Work out the finished part from the listing and answer in its coordinate system (mm). A direction names the side the tool comes from. Give positions to 0.01 mm unless a question says otherwise; leave off trailing zeros. Write each loop counter-clockwise with the first axis right and the second up, starting at its lowest first coordinate (ties: lowest second). Pieces come first, ordered by that corner, then holes.
1) A tool of negligible diameter and unlimited length cuts with its end or side. For faces 4 (the face through (9.1, 3.4, -3.3)), 5 (the face through (-0.1, 8.3, 6.2)), from which of +Z, -Z, +X, -X, +Y, -Y can it reach the whole face along a straight path? Write none if from no direction.
2) Find section D-D (x = 6.5). Determine the outline of the cut face in (y, z), plus the area to 3 significant figures.
3) Find section B-B (z = 0). Determine the outline of the cut face in (x, y) (3 decimals), plus the area to 3 significant figures.
4) Straight lines are drawn through the part: probe 1 along Z at (x, y) = (0, 6.5) (3 decimals); probe 2 along Y at (x, z) = (12.75, -2.25); probe 3 along X at (y, z) = (4, -0.75). For each, find the intervals that lie inside material, in ascending order.
5) Find section A-A (x = 0). Determine the outline of the cut face in (y, z) (3 decimals).
6) Determine the mould class of faces 1 (the face through (3, 0, 6)), 2 (the face through (-6, 4, 0)), 3 (the face through (-7.559, 5.816, 5.796)) for opening direction Z: pulls with the +Z half, pulls with the -Z half, needs draft (parallel to the pull), parting line crosses it, or undercut.
7) Given pin 1 Ø4 at (y, z) = (3, 5) entering from +X; pin 2 Ø5 at (x, z) = (1, -0.5) entering from +Y; pin 3 Ø3 at (x, z) = (-3, 11) entering from -Y; pin 4 Ø4 at (y, z) = (3.5, -6.5) entering from -X, each flat-ended and moving along its own axis, determine where each tip first touches the part or whether it passes through.
8) Find section C-C (y = 1.25). Determine the outline of the cut face in (x, z).
```python
from build123d import *

# Parameters (mm, degrees)
SKETCH1_R           = 13.9
BOSS_EXTRUDE1_DEPTH = 3.4
SKETCH2_R           = 9.525
BOSS_EXTRUDE2_DEPTH = 4.9
SKETCH3_R           = 6
CUT_EXTRUDE1_DEPTH  = 8.3


with BuildPart() as part:
    # Sketch1 → Boss-Extrude1 (new body)
    with BuildSketch(Plane(origin=(0, 0, 0), x_dir=(1, 0, 0), z_dir=(0, 1, 0))):
        Circle(SKETCH1_R)
    extrude(amount=BOSS_EXTRUDE1_DEPTH)

    # Sketch2 → Boss-Extrude2 (add)
    with BuildSketch(Plane(origin=(0, 3.4, 0), x_dir=(1, 0, 0), z_dir=(0, 1, 0))):
        Circle(SKETCH2_R)
    extrude(amount=BOSS_EXTRUDE2_DEPTH)

    # Sketch3 → Cut-Extrude1 (cut)
    with BuildSketch(Plane.XZ):
        Circle(SKETCH3_R)
    extrude(amount=-CUT_EXTRUDE1_DEPTH, mode=Mode.SUBTRACT)


solid = part.part
```
Results:
1. face 4: +Y
1. face 5: +Z, -Z, +X, -X, +Y
2. outline: (0, -12.29) - (3.4, -12.29) - (3.4, -6.96) - (8.3, -6.96) - (8.3, 6.96) - (3.4, 6.96) - (3.4, 12.29) - (0, 12.29) - close
2. area: 152 mm2
3. outline: (-13.9, 0) - (-6, 0) - (-6, 8.3) - (-9.525, 8.3) - (-9.525, 3.4) - (-13.9, 3.4) - close; (6, 0) - (13.9, 0) - (13.9, 3.4) - (9.525, 3.4) - (9.525, 8.3) - (6, 8.3) - close
3. area: 88.3 mm2
4. probe 1: z = -9.525 to -6, 6 to 9.525
4. probe 2: y = 0 to 3.4
4. probe 3: x = -9.5 to -5.95, 5.95 to 9.5
5. outline: (0, -13.9) - (3.4, -13.9) - (3.4, -9.525) - (8.3, -9.525) - (8.3, -6) - (0, -6) - close; (0, 6) - (8.3, 6) - (8.3, 9.525) - (3.4, 9.525) - (3.4, 13.9) - (0, 13.9) - close
6. face 1: needs draft
6. face 2: undercut
6. face 3: parting line crosses it
7. pin 1: stops at x = 13.57
7. pin 2: passes through
7. pin 3: stops at y = 0
7. pin 4: stops at x = -13.15
8. outline: circle Ø27.8 at (0, 0); hole circle Ø12 at (0, 0)
